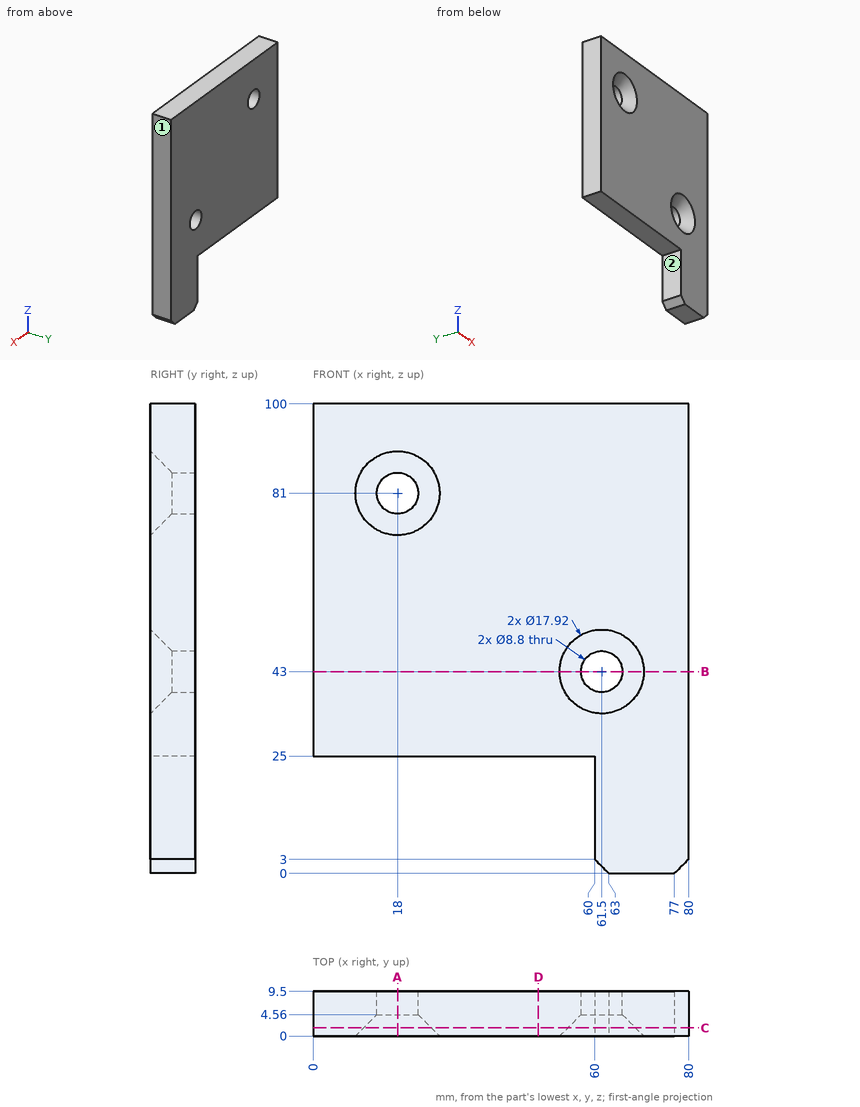
For this review, use the dimensioned drawing (mm, ordinates from the lowest corner) and the shaded views. A direction names the side the tool comes from. Coordinates: 2 decimals unless noted, no trailing zeros. Loops run counter-clockwise (first coordinate to the right, second up) from the corner with the lowest first, then second, coordinate; pieces in that order, holes last. Notation, with made-up numbers: (76, 44) -> (134, 44) arc R24 ccw to (134, 62) -> close; hole circle Ø9 at (84, 59). An arc over 180 degrees is marked (long way). Write each question's results on one line, items separated by ' | '.
Q1. Machinability: for the marked faces 1 and 2, which of the approach directions +Z, -Z, +X, -X, +Y, -Y give a long, thin tool a straight path to every point of the face, cutting with its end or side? Answer none if there is none.
Taken from the geometry:
face 1: +Z, -Z, +X, +Y, -Y | face 2: -Z, -X, +Y, -Y
Q2. For pin 1 Ø2 at (x, y) = (24.5, 6) entering from -Z; pin 2 Ø3 at (y, z) = (6, 15.5) entering from -X, all flat-tipped, find the tip position at first contact; note any pin that passes through.
Taken from the geometry:
pin 1: z = 25 | pin 2: x = 60
Q3. Add section D-D, the plane x = 48. State the section outline as (y, z) points.
Taken from the geometry:
outline: (0, 25) -> (9.5, 25) -> (9.5, 100) -> (0, 100) -> close
Q4. Add section C-C, the plane y = 1.75. State the section outline as (x, z) points.
Taken from the geometry:
outline: (0, 25) -> (60, 25) -> (60, 3) -> (63, 0) -> (77, 0) -> (80, 3) -> (80, 100) -> (0, 100) -> close; hole circle Ø14.42 at (18, 81); hole circle Ø14.42 at (61.5, 43)
Q5. Add section B-B, the plane z = 43. State the section outline as (x, y) points.
Taken from the geometry:
outline: (0, 0) -> (52.54, 0) -> (57.1, 4.56) -> (57.1, 9.5) -> (0, 9.5) -> close; (65.9, 4.56) -> (70.46, 0) -> (80, 0) -> (80, 9.5) -> (65.9, 9.5) -> close
Q6. Add section A-A, the plane x = 18. State the section outline as (y, z) points, then the cut area to 3 significant figures.
Taken from the geometry:
outline: (0, 25) -> (9.5, 25) -> (9.5, 76.6) -> (4.56, 76.6) -> (0, 72.04) -> close; (0, 89.96) -> (4.56, 85.4) -> (9.5, 85.4) -> (9.5, 100) -> (0, 100) -> close | area: 608 mm²
Q7. To check wall thickness, follow line 1 along X through (y, z) = (7.65, 81); line 2 along Z through (x, y) = (18, 6.1); line 3 along X through (y, z) = (8.75, 43). State the ranges of each line that lie inside material, in increasing order. Write a range as [from, to].
Taken from the geometry:
line 1: [0, 13.6], [22.4, 80] | line 2: [25, 76.6], [85.4, 100] | line 3: [0, 57.1], [65.9, 80]
